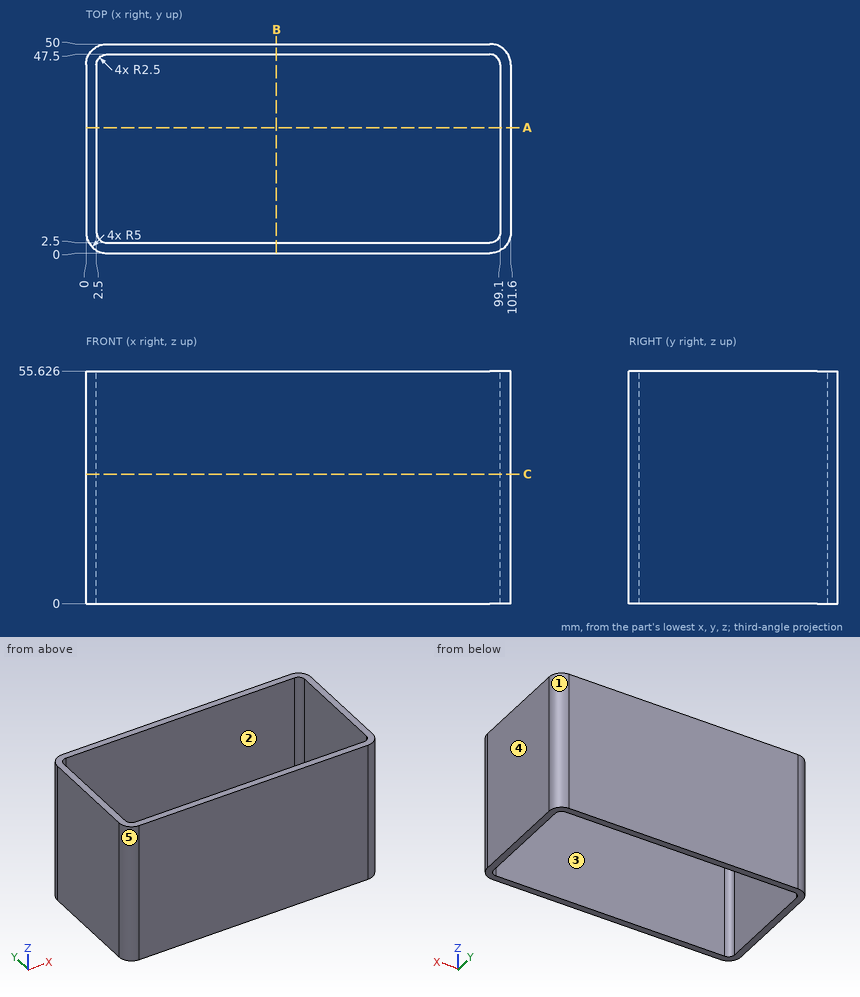
Geometry check sheet. Reference: drawing and pictorial views, mm from the part's lowest x, y, z. A direction names the side the tool comes from. Coordinates: 2 decimals unless noted, no trailing zeros. Order: outer loops, then holes, each group sorted by start corner. A loop starts at its lowest first (then second) coordinate and runs counter-clockwise, first axis right, second up. Notation, with made-up numbers: (-32.75, -31.75) - (-3.75, -31.75) arc R19 ccw to (-3.75, -5.75) - close; hole circle Ø3 at (22, 48). An arc over 180 degrees is marked (long way). One line per item, written item: value.
(1) Sectioned sample at A-A (y = 30). Enter the section's corners in (x, z), and give its area (3 significant figures).
Data:
outline: (0, 0) - (2.5, 0) - (2.5, 55.63) - (0, 55.63) - close; (99.1, 0) - (101.6, 0) - (101.6, 55.63) - (99.1, 55.63) - close
area: 278 mm^2
(2) Sectioned sample at C-C (z = 31). Enter the section's corners in (x, y), and give its area (3 significant figures).
Data:
outline: (0, 5) arc R5 ccw to (5, 0) - (96.6, 0) arc R5 ccw to (101.6, 5) - (101.6, 45) arc R5 ccw to (96.6, 50) - (5, 50) arc R5 ccw to (0, 45) - close; hole (2.5, 5) arc R2.5 ccw to (5, 2.5) - (96.6, 2.5) arc R2.5 ccw to (99.1, 5) - (99.1, 45) arc R2.5 ccw to (96.6, 47.5) - (5, 47.5) arc R2.5 ccw to (2.5, 45) - close
area: 717 mm^2
(3) Sectioned sample at B-B (x = 45.5). Enter the section's corners in (y, z).
Data:
outline: (0, 0) - (2.5, 0) - (2.5, 55.63) - (0, 55.63) - close; (47.5, 0) - (50, 0) - (50, 55.63) - (47.5, 55.63) - close
(4) Access from +Z, -Z, +X, -X, +Y, -Y to the whole of each face (thin tool, end or side, straight path). Record for the marked faces 1 and 2.
Data:
face 1: +Z, -Z, +X, +Y
face 2: +Z, -Z
(5) Release check for a two-part mould opening along Y. For the marked faces 3, 4 and 5 record: +Y half, -Y half, draft (parallel to the pull), parting line (faces both ways), or undercut.
Data:
face 3: undercut
face 4: draft
face 5: -Y half
(6) Thickness scan on probe 1 along X at (y, z) = (12, 20.5); probe 2 along Y at (x, z) = (72, 27.5); probe 3 along X at (y, z) = (3, 40.5). Record the ranges inside material, lowest first. Write a range as from..to.
Data:
probe 1: x = 0..2.5, 99.1..101.6
probe 2: y = 0..2.5, 47.5..50
probe 3: x = 0.42..3.5, 98.1..101.18
